Check sheet for the drawn part. Datum: minimum x, y, z corner. Units: mm. Coordinates: 2 decimals unless noted, no trailing zeros. Order: outer loops, then holes, each group sorted by start corner. A loop starts at its lowest first (then second) coordinate and runs counter-clockwise, first axis right, second up.
1. Cross-section at B-B (x = 43). Enter the section's corners in (y, z), then the cut area to 3 significant figures.
2. Cross-section at D-D (y = 25). Enter the section's corners in (x, z).
3. Cross-section at C-C (z = 0.6). Enter the section's corners in (x, y), then the cut area to 3 significant figures.
4. Gauge pin test, flat ends, axial feed: pin 1 Ø1.5 at (x, z) = (49, 0.5) entering from +Y; pin 2 Ø1.5 at (x, z) = (13, 2) entering from -Y. Record the tip position at first contact, or that the pin passes through.
5. Cross-section at A-A (y = 43). Enter the section's corners in (x, z), then the cut area to 3 significant figures.
6. Thickness scan on line 1 (Y direction, x = 43, z = 2.7); line 2 (Y direction, x = 12, z = 2.75); line 3 (Y direction, x = 51, z = 2.05). Record the ranges inside material, lowest first.
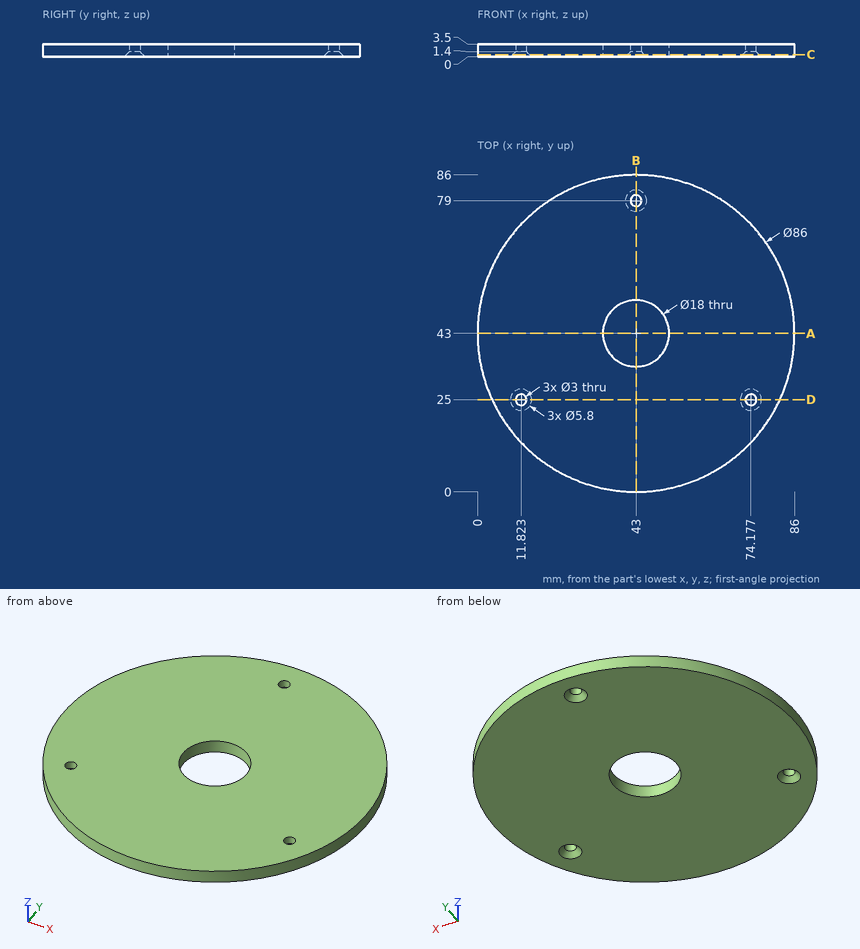
Data:
1. outline: (0, 0) - (34, 0) - (34, 3.5) - (0, 3.5) - close; (52, 0) - (76.1, 0) - (77.5, 1.4) - (77.5, 3.5) - (52, 3.5) - close; (80.5, 1.4) - (81.9, 0) - (86, 0) - (86, 3.5) - (80.5, 3.5) - close
1. area: 226 mm2
2. outline: (3.95, 0) - (8.92, 0) - (10.32, 1.4) - (10.32, 3.5) - (3.95, 3.5) - close; (13.32, 1.4) - (14.72, 0) - (71.28, 0) - (72.68, 1.4) - (72.68, 3.5) - (13.32, 3.5) - close; (75.68, 1.4) - (77.08, 0) - (82.05, 0) - (82.05, 3.5) - (75.68, 3.5) - close
3. outline: circle Ø86 at (43, 43); hole circle Ø4.6 at (11.82, 25); hole circle Ø18 at (43, 43); hole circle Ø4.6 at (43, 79); hole circle Ø4.6 at (74.18, 25)
3. area: 5,500 mm2
4. pin 1: stops at y = 85.68
4. pin 2: stops at y = 11.48
5. outline: (0, 0) - (34, 0) - (34, 3.5) - (0, 3.5) - close; (52, 0) - (86, 0) - (86, 3.5) - (52, 3.5) - close
5. area: 238 mm2
6. line 1: y = 0 to 34, 52 to 77.5, 80.5 to 86
6. line 2: y = 13.2 to 23.51, 26.49 to 72.8
6. line 3: y = 0.75 to 38.88, 47.12 to 85.25
